Autodesk Inventor part; units mm, degrees
ref_plane "YZ Plane" through (0, 0, 0) normal (1, 0, 0) x (0, 1, 0)
ref_plane "XZ Plane" through (0, 0, 0) normal (0, 1, 0) x (-1, 0, 0)
ref_plane "XY Plane" through (0, 0, 0) normal (0, 0, 1) x (1, 0, 0)
sketch "Sketch1" plane through (0, 0, 0) normal (0, 0, 1) x (1, 0, 0)
  line L0 (0, 0) -> (212.725, 0)
  line L1 (212.725, 0) -> (212.725, 101.6)
  line L2 (212.725, 101.6) -> (0, 101.6)
  line L3 (0, 101.6) -> (0, 0)
  dimension "d0" = 212.725
  dimension "d1" = 101.6
extrude "Extrusion1" add sketch "Sketch1" along normal blind 3
sketch "Sketch2" plane through (0, 0, 3) normal (0, 0, 1) x (1, 0, 0)
  line L0 (6.35, 0) -> (206.375, 0)
  line L1 (206.375, 0) -> (206.375, 57.15)
  line L2 (206.375, 57.15) -> (6.35, 57.15)
  line L3 (6.35, 57.15) -> (6.35, 0)
  line L4 (0, 0) -> (212.725, 0)
  line L5 (212.725, 0) -> (212.725, 101.6)
  line L6 (212.725, 101.6) -> (0, 101.6)
  line L7 (0, 101.6) -> (0, 0)
  dimension "d4" = 57.15
  dimension "d9" = 6.35
  dimension "d10" = 6.35
extrude "Extrusion2" cut sketch "Sketch2" against normal blind 3.5 contours L3 L2 L1 L0
sketch "Sketch3" plane through (0, 0, 3) normal (0, 0, 1) x (1, 0, 0)
  line L0 (206.375, 57.15) -> (206.375, 0)
  line L1 (206.375, 0) -> (212.725, 0)
  line L2 (212.725, 0) -> (212.725, 101.6)
  line L3 (212.725, 101.6) -> (0, 101.6)
  line L4 (0, 101.6) -> (0, 0)
  line L5 (0, 0) -> (6.35, 0)
  line L6 (6.35, 0) -> (6.35, 57.15)
  line L7 (6.35, 57.15) -> (206.375, 57.15)
  line L8 (0, 0) -> (3, 0)
  line L9 (3, 0) -> (3, 12.5984)
  line L10 (3, 12.5984) -> (0, 12.5984)
  line L11 (0, 12.5984) -> (0, 0)
  line L12 (3, 25.4) -> (3, 37.9984)
  line L13 (3, 37.9984) -> (0, 37.9984)
  line L14 (0, 37.9984) -> (0, 25.4)
  line L15 (0, 25.4) -> (3, 25.4)
  line L16 (3, 50.8) -> (3, 63.3984)
  line L17 (3, 63.3984) -> (0, 63.3984)
  line L18 (0, 63.3984) -> (0, 50.8)
  line L19 (0, 50.8) -> (3, 50.8)
  line L20 (3, 76.2) -> (3, 88.7984)
  line L21 (3, 88.7984) -> (0, 88.7984)
  line L22 (0, 88.7984) -> (0, 76.2)
  line L23 (0, 76.2) -> (3, 76.2)
  line L24 (3, 101.6) -> (3, 114.1984)
  line L25 (3, 114.1984) -> (0, 114.1984)
  line L26 (0, 114.1984) -> (0, 101.6)
  line L27 (0, 101.6) -> (3, 101.6)
  dimension "d11" = 12.5984
  dimension "d12" = 3
  dimension "d15" = 25.4
extrude "Extrusion3" cut sketch "Sketch3" against normal blind 3 contours L5 L4 L10 L9 | L3 L26 L25 L24 | L21 L20 L23 L4 | L4 L13 L12 L15 | L17 L16 L19 L4
properties part number "PCBWall"
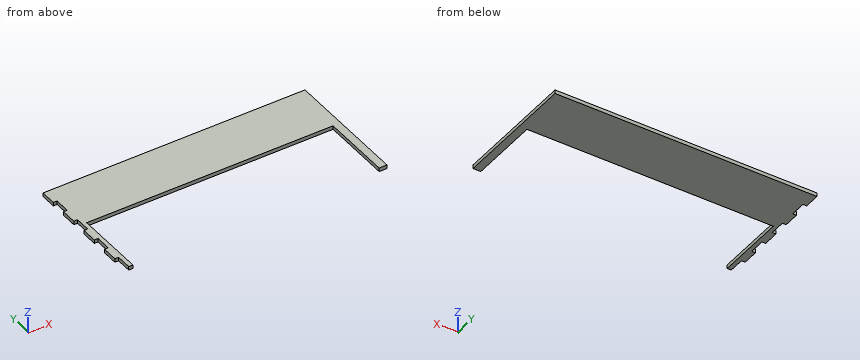
Can you work these out from the model? Positions are in its coordinate system, mm. Coordinates: 2 decimals unless noted, no trailing zeros. Loops run counter-clockwise (first coordinate to the right, second up) from the corner with the lowest first, then second, coordinate; pieces in that order, holes last.
1) Imagine slicing it at C-C on x = 44. List the corners of the cut face in (y, z) for me.
2) I need wall thicknesses on probe 1 along X at (y, z) = (47, 1.65) (3 decimals); probe 2 along X at (y, z) = (32.5, 0.2) (3 decimals); probe 3 along Y at (x, z) = (188, 2.05). Which ranges of each line are inside material? Lowest first, please.
3) Imagine slicing it at B-B on z = 1.8. List the corners of the cut face in (x, y) for me (3 decimals).
4) Imagine slicing it at A-A on y = 41. List the corners of the cut face in (x, z) for me (3 decimals).
5) For pin 1 (1.5 mm diameter, centred on y = 17, z = 2, fed in from -X); pin 2 (1.5 mm diameter, centred on x = 1, z = 1, fed in from -Y); pin 3 (1.5 mm diameter, centred on y = 9.5, z = 2, fed in from -X); pin 4 (1.5 mm diameter, centred on x = 83, z = 1, fed in from -Y), each with a flat end and sliding along its axis, tell me the tip position at first contact or that it passes through.
Completed:
1. outline: (57.15, 0) - (101.6, 0) - (101.6, 3) - (57.15, 3) - close
2. probe 1: x = 0 to 6.35, 206.375 to 212.725
2. probe 2: x = 3 to 6.35, 206.375 to 212.725
2. probe 3: y = 57.15 to 101.6
3. outline: (0, 12.598) - (3, 12.598) - (3, 0) - (6.35, 0) - (6.35, 57.15) - (206.375, 57.15) - (206.375, 0) - (212.725, 0) - (212.725, 101.6) - (0, 101.6) - (0, 88.798) - (3, 88.798) - (3, 76.2) - (0, 76.2) - (0, 63.398) - (3, 63.398) - (3, 50.8) - (0, 50.8) - (0, 37.998) - (3, 37.998) - (3, 25.4) - (0, 25.4) - close
4. outline: (0, 0) - (6.35, 0) - (6.35, 3) - (0, 3) - close; (206.375, 0) - (212.725, 0) - (212.725, 3) - (206.375, 3) - close
5. pin 1: stops at x = 0
5. pin 2: stops at y = 12.6
5. pin 3: stops at x = 3
5. pin 4: stops at y = 57.15
